Build history of the part. All positions in model axes, mm. Round coordinates to 2 decimals unless told otherwise and drop trailing zeros. Write each loop counter-clockwise with the first axis right and the second up, starting at its lowest first coordinate (ties: lowest second). Pieces come first, ordered by that corner, then holes. Notation, with made-up numbers: M -32.5,3.5 L -7.5,3.5 A11 ccw -7.5,15.5 Z; hole C 18.25,32.5 d10. An arc over 180 degrees is marked long. Write item = value, one per line.
from build123d import *

# Parameters (mm, degrees)
CROQUIS1_W                = 50
CROQUIS1_H                = 50
SALIENTE_EXTRUIR1_DEPTH   = 625
SALIENTE_EXTRUIR1_2_DEPTH = 625
SALIENTE_EXTRUIR1_3_DEPTH = 625
SALIENTE_EXTRUIR1_4_DEPTH = 625
CROQUIS2_W                = 90
CROQUIS2_H                = 90
SALIENTE_EXTRUIR2_DEPTH   = 50
CROQUIS4_W                = 50
CROQUIS4_H                = 50
SALIENTE_EXTRUIR3_DEPTH   = 853
SALIENTE_EXTRUIR4_DEPTH   = 50


with BuildPart() as part:
    # Croquis1 → Saliente-Extruir1 (new body)
    with BuildSketch(Plane(origin=(0, 0, 0), x_dir=(1, 0, 0), z_dir=(0, 1, 0))):
        with Locations((-307.842712475, 307.842712475)):
            Rectangle(CROQUIS1_W, CROQUIS1_H)
    extrude(amount=-SALIENTE_EXTRUIR1_DEPTH)



with BuildPart() as body_2:
    # Croquis1 → Saliente-Extruir1 2 (new body)
    with BuildSketch(Plane(origin=(0, 0, 0), x_dir=(1, 0, 0), z_dir=(0, 1, 0))):
        with Locations((307.842712475, 307.842712475)):
            Rectangle(CROQUIS1_W, CROQUIS1_H)
    extrude(amount=-SALIENTE_EXTRUIR1_2_DEPTH)


with BuildPart() as body_3:
    # Croquis1 → Saliente-Extruir1 3 (new body)
    with BuildSketch(Plane(origin=(0, 0, 0), x_dir=(1, 0, 0), z_dir=(0, 1, 0))):
        with Locations((-307.842712475, -307.842712475)):
            Rectangle(CROQUIS1_W, CROQUIS1_H)
    extrude(amount=-SALIENTE_EXTRUIR1_3_DEPTH)


with BuildPart() as body_4:
    # Croquis1 → Saliente-Extruir1 4 (new body)
    with BuildSketch(Plane(origin=(0, 0, 0), x_dir=(1, 0, 0), z_dir=(0, 1, 0))):
        with Locations((307.842712475, -307.842712475)):
            Rectangle(CROQUIS1_W, CROQUIS1_H)
    extrude(amount=-SALIENTE_EXTRUIR1_4_DEPTH)


with BuildPart() as part_1:
    add(part.part)

    add(body_2.part)  # Saliente-Extruir2 merges body 2

    add(body_3.part)  # Saliente-Extruir2 merges body 3

    add(body_4.part)  # Saliente-Extruir2 merges body 4
    # Croquis2 → Saliente-Extruir2 (add)
    with BuildSketch(Plane.XZ.offset(625)):
        with Locations((-307.360997504, 305.1451107)):
            Rectangle(CROQUIS2_W, CROQUIS2_H)
        with Locations((307.360997504, 305.1451107)):
            Rectangle(CROQUIS2_W, CROQUIS2_H)
        with Locations((307.360997504, -305.1451107)):
            Rectangle(CROQUIS2_W, CROQUIS2_H)
        with Locations((-307.360997504, -305.1451107)):
            Rectangle(CROQUIS2_W, CROQUIS2_H)
    extrude(amount=SALIENTE_EXTRUIR2_DEPTH)

    # Croquis4 → Saliente-Extruir3 (add)
    with BuildSketch(Plane.XZ.offset(675)):
        with Locations((-307.842712475, 307.842712475)):
            Rectangle(CROQUIS4_W, CROQUIS4_H)
        with Locations((-307.842712475, -307.842712475)):
            Rectangle(CROQUIS4_W, CROQUIS4_H)
        with Locations((307.842712475, 307.842712475)):
            Rectangle(CROQUIS4_W, CROQUIS4_H)
        with Locations((307.842712475, -307.842712475)):
            Rectangle(CROQUIS4_W, CROQUIS4_H)
    extrude(amount=SALIENTE_EXTRUIR3_DEPTH)

    # Croquis6 → Saliente-Extruir4 (add)
    with BuildSketch(Plane(origin=(0, -800, 0), x_dir=(1, 0, 0), z_dir=(0, 1, 0))):
        Polygon((332.842712475, 282.842712475), (332.842712475, -332.842712475), (282.842712475, -332.842712475), (282.842712475, -282.842712475), (282.842712475, 157.157287525), (-282.842712475, 157.157287525), (-282.842712475, -282.842712475), (-282.842712475, -332.842712475), (-332.842712475, -332.842712475), (-332.842712475, 282.842712475), (-282.842712475, 282.842712475), (-282.842712475, 207.157287525), (282.842712475, 207.157287525), (282.842712475, 282.842712475), align=None)
    extrude(amount=-SALIENTE_EXTRUIR4_DEPTH)


solid = part_1.part
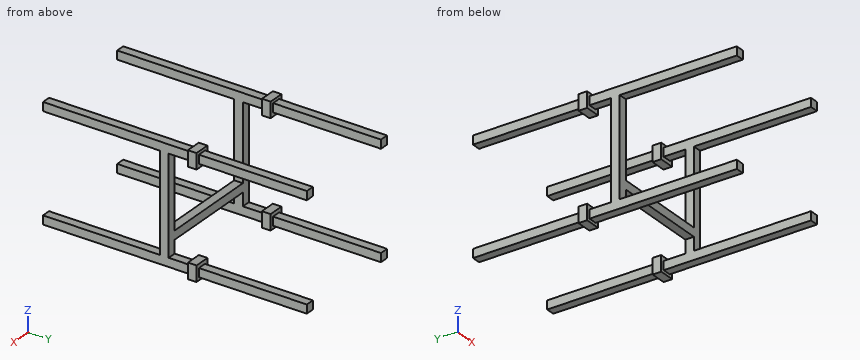
1. Band-saw the part on A-A (y = -150.5). List the corners of the cut face in (x, z).
Responses:
outline = M -332.84,-332.84 L -282.84,-332.84 L -282.84,-282.84 L -332.84,-282.84 Z; M -332.84,282.84 L -282.84,282.84 L -282.84,332.84 L -332.84,332.84 Z; M 282.84,-332.84 L 332.84,-332.84 L 332.84,-282.84 L 282.84,-282.84 Z; M 282.84,282.84 L 332.84,282.84 L 332.84,332.84 L 282.84,332.84 Z
2. Probe probe 1 along Z at (x, y) = (-295, -1224.5); probe 2 along Y at (x, z) = (-314, 131). List the from-to ranges inside material, lowest first.
Responses:
probe_1 = -332.84 to -282.84, 282.84 to 332.84
probe_2 = -850 to -800
3. Band-saw the part on B-B (z = -132). List the corners of the cut face in (x, y).
Responses:
outline = M -332.84,-850 L -282.84,-850 L -282.84,-800 L -332.84,-800 Z; M 282.84,-850 L 332.84,-850 L 332.84,-800 L 282.84,-800 Z
4. Band-saw the part on D-D (x = -165). List the corners of the cut face in (y, z), plus the area to 3 significant figures.
Responses:
outline = M -850,-207.16 L -800,-207.16 L -800,-157.16 L -850,-157.16 Z
area = 2,500 mm²
5. Flat gauge pins, fed straight in: pin 1 (15 mm diameter, centred on x = 310.5, y = -412, fed in from -Z); pin 2 (15 mm diameter, centred on x = -295.5, y = -256.5, fed in from +Z); pin 3 (8 mm diameter, centred on x = -124, z = -168.5, fed in from +Y). Where does each tip first touch, or does it go through?
Responses:
pin_1 = -332.84
pin_2 = 332.84
pin_3 = -800
6. Band-saw the part on C-C (z = -301.5). List the corners of the cut face in (x, y), plus the area to 3 significant figures.
Responses:
outline = M -352.36,-675 L -332.84,-675 L -332.84,-1528 L -282.84,-1528 L -282.84,-675 L -262.36,-675 L -262.36,-625 L -282.84,-625 L -282.84,0 L -332.84,0 L -332.84,-625 L -352.36,-625 Z; M 262.36,-675 L 282.84,-675 L 282.84,-1528 L 332.84,-1528 L 332.84,-675 L 352.36,-675 L 352.36,-625 L 332.84,-625 L 332.84,0 L 282.84,0 L 282.84,-625 L 262.36,-625 Z
area = 157,000 mm²
